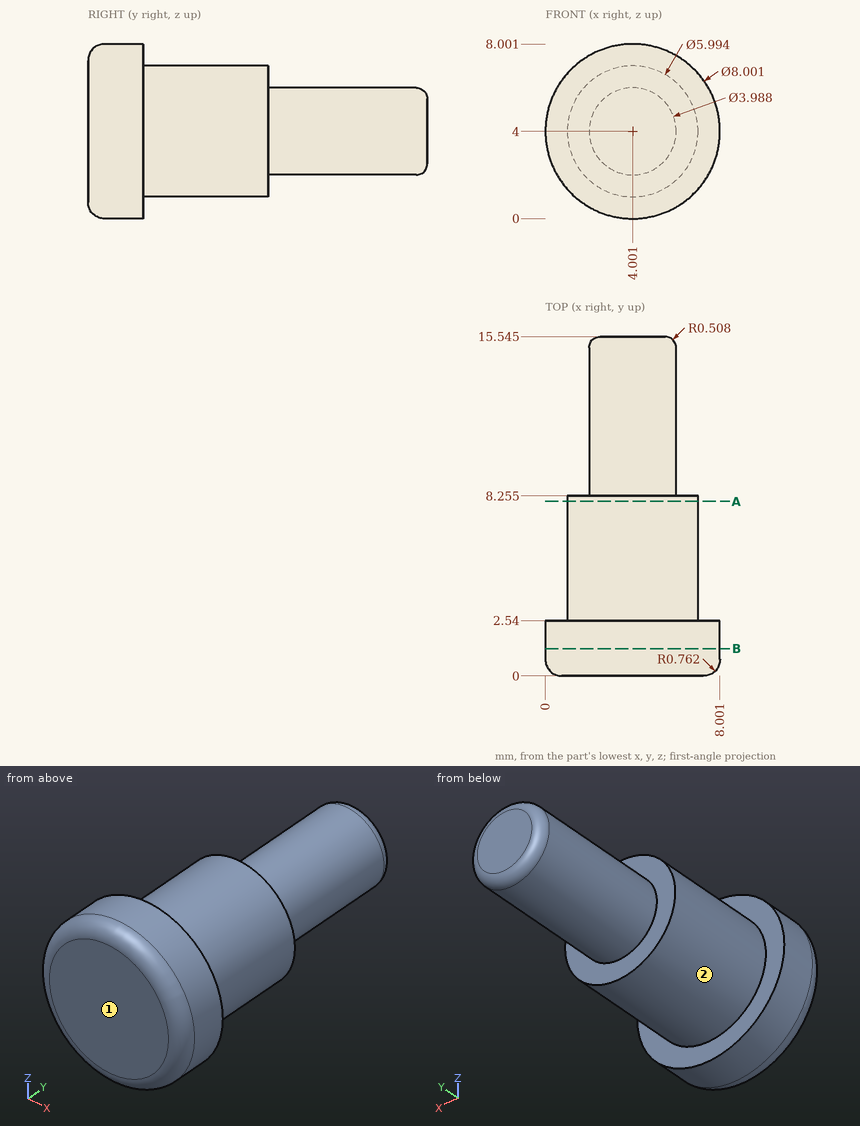
Could you check a few things on this drawing? It's one solid part, dimensions in mm from its lowest x, y, z. A direction names the side the tool comes from. Round coordinates to 2 decimals unless told otherwise and drop trailing zeros. Write each loop counter-clockwise with the first axis right and the second up, starting at its lowest first coordinate (ties: lowest second). Pieces come first, ordered by that corner, then holes. Notation, with made-up numbers: (10, -27.5) -> (62, -27.5) arc R19 ccw to (62, -5.5) -> close; hole circle Ø7 at (-11.75, 84). An arc over 180 degrees is marked (long way). Use one line per item in the form item = value. Start each with the question number.
Q1. If I drill on probe 1 along Y at (x, z) = (5, 1); probe 2 along Y at (x, z) = (3.25, 2) (1 decimal); probe 3 along Z at (x, y) = (4, 7.75), over which ranges is the centre line in solid material (lowest first)? Write a range as [from, to].
Q2. Imagine slicing it at A-A (y = 8). Please give me the cut outline in (x, z) (1 decimal).
Q3. Which directions (+Z, -Z, +X, -X, +Y, -Y) give clear straight access to the entire face, cutting with the end or side of a thin tool? Please do the marked faces 1 and 2.
Q4. Imagine slicing it at B-B (y = 1.25). Please give me the cut outline in (x, z), then the cut area to 3 significant figures.
Q5. I'm going to push flat-ended pins straight in: P1, Ø3, axis at x = 7, y = 9, coming from the +Z side; P2, Ø4, axis at y = 6.5, z = 3, coming from the +X side; P3, Ø1.5, axis at x = 3, z = 5.5, coming from the -Y side. Where does each tip first touch, or does it pass through?
Worked out:
q1.probe_1 = [0, 2.54]
q1.probe_2 = [0, 8.3]
q1.probe_3 = [1, 7]
q2.outline = circle Ø6 at (4, 4)
q3.face_1 = +Z, -Z, +X, -X, -Y
q3.face_2 = +Y
q4.outline = circle Ø8 at (4, 4)
q4.area = 50.3 mm^2
q5.P1 = 6.47
q5.P2 = 7
q5.P3 = 0
